Autodesk Fusion 360 part; units mm, degrees
sketch "スケッチ1" plane through (0, 0, 0) normal (0, 0, 1) x (1, 0, 0)
  circle A0 centre (0, 0) radius 21
  dimension "d1" = 42
extrude "押し出し1" add sketch "スケッチ1" along normal blind 4.5
sketch "スケッチ2" plane through (0, 0, 4.5) normal (0, 0, 1) x (-1, 0, 0)
  circle A0 centre (0, 0) radius 21
  circle A1 centre (0, 0) radius 12.3
  dimension "d4" = 24.6
extrude "押し出し2" add sketch "スケッチ2" along normal blind 5 contours A1
sketch "スケッチ3" plane through (0, 0, 9.5) normal (0, 0, 1) x (-1, 0, 0)
  circle A0 centre (0, 0) radius 4.15
  dimension "d7" = 8.3
extrude "押し出し3" cut sketch "スケッチ3" against normal blind 4.2
sketch "スケッチ4" plane through (0, 0, 0) normal (0, 0, -1) x (1, 0, 0)
  circle A0 centre (0, 0) radius 21
  circle A1 centre (0, 0) radius 8
  circle A2 centre (0, -8) radius 1.15
  circle A3 centre (8, 0) radius 1.15
  circle A4 centre (0, 8) radius 1.15
  circle A5 centre (-8, 0) radius 1.15
  dimension "d10" = 16
  dimension "d11" = 2.3
  dimension "d12" = 2.3
  dimension "d13" = 2.3
  dimension "d14" = 2.3
extrude "押し出し4" cut sketch "スケッチ4" against normal through all contours A1 A3 | A1 A3 | A1 A4 | A1 A4 | A1 A2 | A1 A2 | A1 A5 | A1 A5
sketch "スケッチ5" plane through (0, 0, 0) normal (0, 0, -1) x (1, 0, 0)
  circle A0 centre (8, 0) radius 1.15
  circle A1 centre (0, 8) radius 1.15
  circle A2 centre (0, -8) radius 1.15
  circle A3 centre (-8, 0) radius 1.15
  circle A4 centre (0, 0) radius 21
  line L0 (12, -6) -> (-12, -6)
  line L1 (-12, -6) -> (-12, 6)
  line L2 (-12, 6) -> (12, 6)
  line L3 (12, 6) -> (12, -6)
  circle A5 centre (12, -6) radius 1.4
  circle A6 centre (-12, -6) radius 1.4
  circle A7 centre (12, 6) radius 1.4
  circle A8 centre (-12, 6) radius 1.4
  dimension "d16" = 24
  dimension "d17" = 12
  dimension "d18" = 12
  dimension "d19" = 6
  dimension "d20" = 2.8
  dimension "d21" = 2.8
  dimension "d22" = 2.8
  dimension "d23" = 2.8
extrude "押し出し5" cut sketch "スケッチ5" against normal through all contours L0 L1 A6 | L0 L1 A6 | L0 L3 A5 | L0 L3 A5 | L1 L2 A8 | L1 L2 A8 | L2 L3 A7 | L2 L3 A7
sketch "スケッチ6" plane through (0, 0, 0) normal (0, 0, -1) x (1, 0, 0)
  circle A0 centre (0, 0) radius 21
  circle A1 centre (-8, 0) radius 1.15
  circle A2 centre (0, -8) radius 1.15
  circle A3 centre (0, 8) radius 1.15
  circle A4 centre (8, 0) radius 1.15
  circle A5 centre (-12, 6) radius 1.4
  circle A6 centre (12, -6) radius 1.4
  circle A7 centre (-12, -6) radius 1.4
  circle A8 centre (12, 6) radius 1.4
  circle A9 centre (0, -8) radius 2
  circle A10 centre (8, 0) radius 2
  circle A11 centre (-8, 0) radius 2
  circle A12 centre (0, 8) radius 2
  dimension "d25" = 4
  dimension "d26" = 4
  dimension "d27" = 4
  dimension "d28" = 4
extrude "押し出し6" cut sketch "スケッチ6" against normal blind 8 contours A9 | A10 | A11 | A12
sketch "スケッチ7" plane through (0, 0, 9.5) normal (0, 0, 1) x (-1, 0, 0)
  arc A0 (-11.3392, 4.7658) -> (-10.6161, 6.2119) centre (-12, 6) ccw
  arc A1 (-11.3392, 4.7658) -> (-11.3392, -4.7658) centre (0, 0) ccw
  arc A2 (-10.6161, -6.2119) -> (-11.3392, -4.7658) centre (-12, -6) ccw
  arc A3 (-10.6161, -6.2119) -> (10.6161, -6.2119) centre (0, 0) ccw
  arc A4 (11.3392, -4.7658) -> (10.6161, -6.2119) centre (12, -6) ccw
  arc A5 (11.3392, -4.7658) -> (11.3392, 4.7658) centre (0, 0) ccw
  arc A6 (10.6161, 6.2119) -> (11.3392, 4.7658) centre (12, 6) ccw
  arc A7 (10.6161, 6.2119) -> (-10.6161, 6.2119) centre (0, 0) ccw
  circle A8 centre (-8, 0) radius 1.15
  circle A9 centre (0, 8) radius 1.15
  circle A10 centre (0, -8) radius 1.15
  circle A11 centre (8, 0) radius 1.15
  circle A12 centre (0, 0) radius 4.15
  circle A13 centre (-12, 6) radius 3
  circle A14 centre (-12, -6) radius 3
  circle A15 centre (12, 6) radius 3
  circle A16 centre (12, -6) radius 3
  dimension "d31" = 6
  dimension "d32" = 6
  dimension "d33" = 6
  dimension "d34" = 6
extrude "押し出し7" cut sketch "スケッチ7" against normal blind 7 contours A0 A1 A7 A13 | A0 A1 A7 A13 | A1 A2 A3 A14 | A1 A2 A3 A14 | A5 A6 A7 A15 | A5 A6 A7 A15 | A3 A4 A5 A16 | A3 A4 A5 A16
equation "d18 = d16 / 2"
equation "d19 = d17 / 2"
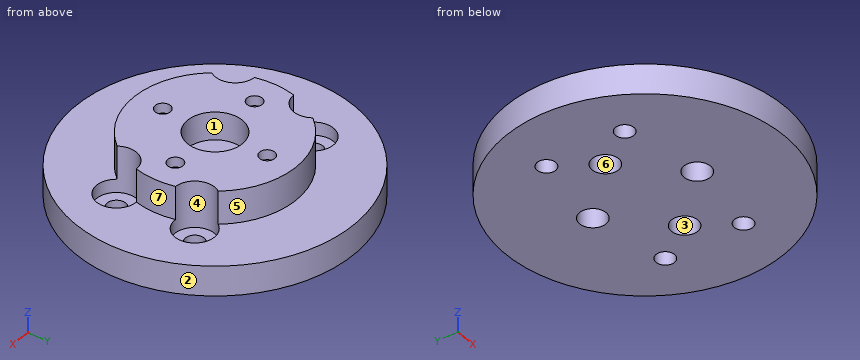
Work out the finished part from the listing and answer in its coordinate system (mm). Face numbers are marked on the shaded views. A direction names the side the tool comes from. Give positions to 0.01 mm unless a question says otherwise; leave off trailing zeros. Loops run counter-clockwise (first coordinate to the right, second up) from the corner with the lowest first, then second, coordinate; pieces in that order, holes last. Notation, with made-up numbers: M 74,59 L 129,59 A19 ccw 129,79 Z; hole C -34,21 d9. An arc over 180 degrees is marked long. One line per item, written item: value. Start each with the question number.
1. Find the intervals of material crossed by probe 1 along X at (y, z) = (0, 8.55); probe 2 along Y at (x, z) = (0, 7.85), in increasing order.
2. Find section C-C (z = 3.75). State how many separate pieces and enclosed holes the cut face has, and give its area (3 significant figures).
3. Which of the six approach directions +Z, -Z, +X, -X, +Y, -Y give full straight-line access (tool end or side, diameter ignored) to the marked faces 1, 2 and 3?
4. Find section D-D (x = 8). Give the vertices of the cut face in (y, z), and give its area (3 significant figures).
5. Each of these flat-tipped pins is pushed along its axis until it touches: P1, Ø2.5, axis at x = 8, y = 0, coming from the -Z side; P2, Ø5, axis at y = -5.5, z = 6, coming from the +X side; P3, Ø4, axis at x = 0.5, z = 1, coming from the +Y side. Where does it stop, or does it pass through?
6. Find section A-A (x = 0). Give the vertices of the cut face in (y, z).
7. Determine the mould class of the marked faces 4, 5, 6 and 7 for opening direction X: released by +X, released by -X, zero draft, split by the parting line, or undercut.
Reported:
1. probe 1: x = -12.3 to -9.15, -6.85 to -4.15, 4.15 to 6.85, 9.15 to 12.3
1. probe 2: y = -12.3 to -10, -6 to -4.15, 4.15 to 6, 10 to 12.3
2. separate pieces: 1
2. enclosed holes: 8
2. area: 1,220 mm²
3. face 1: +Z
3. face 2: +Z, -Z
3. face 3: -Z
4. outline: M -19.42,0 L -2,0 L -2,8 L -1.15,8 L -1.15,9.5 L -9.34,9.5 L -9.34,4.5 L -19.42,4.5 Z; M 1.15,8 L 2,8 L 2,0 L 19.42,0 L 19.42,4.5 L 9.34,4.5 L 9.34,9.5 L 1.15,9.5 Z
4. area: 233 mm²
5. P1: stops at z = 8
5. P2: stops at x = 20.71
5. P3: stops at y = 21
6. outline: M -21,0 L -10,0 L -10,8 L -9.15,8 L -9.15,9.5 L -12.3,9.5 L -12.3,4.5 L -21,4.5 Z; M -6.85,8 L -6,8 L -6,0 L 6,0 L 6,8 L 6.85,8 L 6.85,9.5 L 4.15,9.5 L 4.15,5.3 L -4.15,5.3 L -4.15,9.5 L -6.85,9.5 Z; M 9.15,8 L 10,8 L 10,0 L 21,0 L 21,4.5 L 12.3,4.5 L 12.3,9.5 L 9.15,9.5 Z
7. face 4: undercut
7. face 5: split by the parting line
7. face 6: undercut
7. face 7: released by +X
